Geometry: final body of the model. Coordinates: model frame, mm. Round coordinates to 2 decimals unless told otherwise and drop trailing zeros. Loops run counter-clockwise (first coordinate to the right, second up) from the corner with the lowest first, then second, coordinate; pieces in that order, holes last. Notation, with made-up numbers: M -29,47 L 23,47 A19 ccw 23,84 Z; hole C 77,72.25 d6. An arc over 180 degrees is marked long. Answer as a JSON object with one key per item and string values.
from build123d import *

# Parameters (mm, degrees)
SKETCH1_R           = 110
SKETCH1_R_2         = 90
SKETCH1_R_3         = 1.5
BOSS_EXTRUDE1_DEPTH = 2


with BuildPart() as part:
    # Sketch1 → Boss-Extrude1 (new body)
    with BuildSketch(Plane(origin=(0, 0, 0), x_dir=(1, 0, 0), z_dir=(0, 1, 0))):
        with Locations(Location((0, 0, 0), (0, 0, 270))):
            Circle(SKETCH1_R)
        with Locations(Location((0, 0, 0), (0, 0, 270))):
            Circle(SKETCH1_R_2, mode=Mode.SUBTRACT)
        with Locations(Location((95, 0, 0), (0, 0, 270))):
            Circle(SKETCH1_R_3, mode=Mode.SUBTRACT)
        with Locations(Location((105, 0, 0), (0, 0, 270))):
            Circle(SKETCH1_R_3, mode=Mode.SUBTRACT)
        with Locations(Location((86.602540378, 50, 0), (0, 0, 270))):
            Circle(SKETCH1_R_3, mode=Mode.SUBTRACT)
        with Locations(Location((86.602540378, -50, 0), (0, 0, 270))):
            Circle(SKETCH1_R_3, mode=Mode.SUBTRACT)
        with Locations(Location((52.5, -90.932667397, 0), (0, 0, 270))):
            Circle(SKETCH1_R_3, mode=Mode.SUBTRACT)
        with Locations(Location((47.5, -82.27241336, 0), (0, 0, 270))):
            Circle(SKETCH1_R_3, mode=Mode.SUBTRACT)
        with Locations(Location((0, -100, 0), (0, 0, 270))):
            Circle(SKETCH1_R_3, mode=Mode.SUBTRACT)
        with Locations(Location((-52.5, -90.932667397, 0), (0, 0, 270))):
            Circle(SKETCH1_R_3, mode=Mode.SUBTRACT)
        with Locations(Location((-47.5, -82.27241336, 0), (0, 0, 270))):
            Circle(SKETCH1_R_3, mode=Mode.SUBTRACT)
        with Locations(Location((-86.602540378, -50, 0), (0, 0, 270))):
            Circle(SKETCH1_R_3, mode=Mode.SUBTRACT)
        with Locations(Location((-105, 0, 0), (0, 0, 270))):
            Circle(SKETCH1_R_3, mode=Mode.SUBTRACT)
        with Locations(Location((-95, 0, 0), (0, 0, 270))):
            Circle(SKETCH1_R_3, mode=Mode.SUBTRACT)
        with Locations(Location((-86.602540378, 50, 0), (0, 0, 270))):
            Circle(SKETCH1_R_3, mode=Mode.SUBTRACT)
        with Locations(Location((-52.5, 90.932667397, 0), (0, 0, 270))):
            Circle(SKETCH1_R_3, mode=Mode.SUBTRACT)
        with Locations(Location((-47.5, 82.27241336, 0), (0, 0, 270))):
            Circle(SKETCH1_R_3, mode=Mode.SUBTRACT)
        with Locations(Location((0, 100, 0), (0, 0, 270))):
            Circle(SKETCH1_R_3, mode=Mode.SUBTRACT)
        with Locations(Location((52.5, 90.932667397, 0), (0, 0, 270))):
            Circle(SKETCH1_R_3, mode=Mode.SUBTRACT)
        with Locations(Location((47.5, 82.27241336, 0), (0, 0, 270))):
            Circle(SKETCH1_R_3, mode=Mode.SUBTRACT)
    extrude(amount=BOSS_EXTRUDE1_DEPTH)


solid = part.part
1) Section query A-A (x = -79). Return the cut outline in (y, z), and give its area (3 significant figures).
Results:
{"outline": "M 0,-76.54 L 2,-76.54 L 2,-43.12 L 0,-43.12 Z; M 0,43.12 L 2,43.12 L 2,76.54 L 0,76.54 Z", "area": "134 mm2"}
2) Section query B-B (z = 86.5). Return the cut outline in (x, y), and give its area (3 significant figures).
Results:
{"outline": "M -67.95,0 L -24.85,0 L -24.85,2 L -67.95,2 Z; M 24.85,0 L 67.95,0 L 67.95,2 L 24.85,2 Z", "area": "172 mm2"}
3) Section query C-C (y = 1.25). Count the separate pieces of the cut face and the enclosed holes in it, and give its area (3 significant figures).
Results:
{"separate pieces": "1", "enclosed holes": "19", "area": "12,400 mm2"}
4) Ray query, line 1 (X direction, y = 1.4, z = 0); line 2 (X direction, y = 1.2, z = 50); line 3 (X direction, y = 1.45, z = -2). Return the intervals inside material, ascending.
Results:
{"line 1": "-110 to -106.5, -103.5 to -96.5, -93.5 to -90, 90 to 93.5, 96.5 to 103.5, 106.5 to 110", "line 2": "-97.98 to -88.1, -85.1 to -74.83, 74.83 to 85.1, 88.1 to 97.98", "line 3": "-109.98 to -89.98, 89.98 to 109.98"}
5) Pin query (flat end, axial travel): P1, Ø1.8, axis at x = 52.5, z = 90.93, coming from the -Y side; P2, Ø5, axis at x = 86.6, z = -50, coming from the +Y side; P3, Ø1, axis at y = 1, z = -50.5, coming from the +X side. Return the tip coordinate at first contact, or that it passes through.
Results:
{"P1": "through", "P2": "y = 2", "P3": "x = 97.98"}
6) Pull-direction query (X, two-part tool) for faces 1 (the cylindrical face through (-97.59, 0.99, 50.76)), 2 (the flat face through (90, 0, -9)), 3 (the cylindrical face through (-34.471, 0.986, 83.137)); classes: +X half, -X half, draft (parallel to the pull), parting line (faces both ways), or undercut.
Results:
{"face 1": "parting line", "face 2": "draft", "face 3": "undercut"}
